Source: CAD feature listing. Evaluate the final solid. Frame: model axes, mm. A direction names the side the tool comes from. Round coordinates to 2 decimals unless told otherwise and drop trailing zeros. Loops run counter-clockwise (first coordinate to the right, second up) from the corner with the lowest first, then second, coordinate; pieces in that order, holes last. Notation, with made-up numbers: (-18.5, -31.75) -> (23.5, -31.75) arc R22 ccw to (23.5, -23.75) -> close; hole circle Ø10 at (77.5, 70.5). An arc over 180 degrees is marked (long way). Put each result on its own line as item: value. Start each with the question number.
1. Cut plane C-C (y = 19). Return the cut outline in (x, z).
2. Contact query for flat-ended pins moving along their axis: pin 1 (2 mm diameter, centred on x = -3.65, y = 7.25, fed in from -Z); pin 2 (2.5 mm diameter, centred on y = 0.5, z = 2, fed in from -X); pin 3 (1.5 mm diameter, centred on y = -2.5, z = 4, fed in from -X); pin 4 (1.6 mm diameter, centred on x = 3.65, y = -7.25, fed in from +Z). Output: stop coordinate, or through.
3. Cut plane B-B (y = -17). Return the cut outline in (x, z).
4. Set-up query: faces 1 (the flat face through (130, -2.5, 2)), 2 (the cylindrical face through (-22.495, -0.495, 2.465)). Return all of +Z, -Z, +X, -X, +Y, -Y with unobstructed straight access to the full face (end or side cutting, diameter ignored); none if empty.
5. Material intervals for L1, parallel to Y at x = 3.65, z = 3.8 (3 decimals); L2, parallel to Y at x = 7.25, z = 1.25 (3 decimals); L3, parallel to X at y = -7, z = 2.8, sorted ascending.
6. Draft query along Y for faces 3 (the flat face through (150, 0, 2)), 4 (the flat face through (74, 22.5, 2)), 5 (the flat face through (80, 0, 2)). Return one class per face: pulls with the +Y half, pulls with the -Y half, needs draft (parallel to the pull), parting line crosses it, or undercut.
7. Cut plane A-A (z = 1.45). State how many separate pieces and enclosed holes the cut face has, then the cut area to 3 significant figures.
```python
from build123d import *

# Parameters (mm, degrees)
ESQUISSE1_R        = 3.5
ESQUISSE1_R_2      = 0.875
ESQUISSE1_W        = 10
ESQUISSE1_H        = 5
BOSS_EXTRU_1_DEPTH = 5


with BuildPart() as part:
    # Esquisse1 → Boss.-Extru.1 (new body)
    with BuildSketch(Plane.XY):
        with BuildLine():
            Line((0, 22.5), (150, 22.5))
            Line((150, 22.5), (150, -22.5))
            Line((150, -22.5), (0, -22.5))
            ThreePointArc((0, -22.5), (-22.5, 0), (0, 22.5))
        make_face()
        Circle(ESQUISSE1_R, mode=Mode.SUBTRACT)
        with Locations((7.25, 3.65)):
            Circle(ESQUISSE1_R_2, mode=Mode.SUBTRACT)
        with Locations((7.25, -3.65)):
            Circle(ESQUISSE1_R_2, mode=Mode.SUBTRACT)
        with Locations((3.65, -7.25)):
            Circle(ESQUISSE1_R_2, mode=Mode.SUBTRACT)
        with Locations((-3.65, -7.25)):
            Circle(ESQUISSE1_R_2, mode=Mode.SUBTRACT)
        with Locations((-7.25, -3.65)):
            Circle(ESQUISSE1_R_2, mode=Mode.SUBTRACT)
        with Locations((-7.25, 3.65)):
            Circle(ESQUISSE1_R_2, mode=Mode.SUBTRACT)
        with Locations((-3.65, 7.25)):
            Circle(ESQUISSE1_R_2, mode=Mode.SUBTRACT)
        with Locations((3.65, 7.25)):
            Circle(ESQUISSE1_R_2, mode=Mode.SUBTRACT)
        with Locations((40, 0)):
            Rectangle(ESQUISSE1_W, ESQUISSE1_H, mode=Mode.SUBTRACT)
        with Locations((85, 0)):
            Rectangle(ESQUISSE1_W, ESQUISSE1_H, mode=Mode.SUBTRACT)
        with Locations((130, 0)):
            Rectangle(ESQUISSE1_W, ESQUISSE1_H, mode=Mode.SUBTRACT)
    extrude(amount=BOSS_EXTRU_1_DEPTH)


solid = part.part
```
Solution:
1. outline: (-12.05, 0) -> (150, 0) -> (150, 5) -> (-12.05, 5) -> close
2. pin 1: stops at z = 0
2. pin 2: stops at x = -22.5
2. pin 3: stops at x = -22.43
2. pin 4: passes through
3. outline: (-14.74, 0) -> (150, 0) -> (150, 5) -> (-14.74, 5) -> close
4. face 1: +Z, -Z
4. face 2: +Z, -Z, -X
5. L1: y = -22.5 to -8.125, -6.375 to 6.375, 8.125 to 22.5
5. L2: y = -22.5 to -4.525, -2.775 to 2.775, 4.525 to 22.5
5. L3: x = -21.38 to -4.49, -2.81 to 2.81, 4.49 to 150
6. face 3: needs draft
6. face 4: pulls with the +Y half
6. face 5: undercut
7. separate pieces: 1
7. enclosed holes: 12
7. area: 7,340 mm^2
